Verification items for this drawing (mm, ordinates from the low corner). Coordinates: 2 decimals unless noted, no trailing zeros. Write each loop counter-clockwise with the first axis right and the second up, starting at its lowest first coordinate (ties: lowest second). Pieces come first, ordered by that corner, then holes. Notation, with made-up numbers: (-31.75, 45.5) -> (-10.75, 45.5) arc R18 ccw to (-10.75, 60.5) -> close; hole circle Ø9 at (45, 57). An arc over 180 degrees is marked (long way). Use CSV: the item, a comma, the result in double quotes.
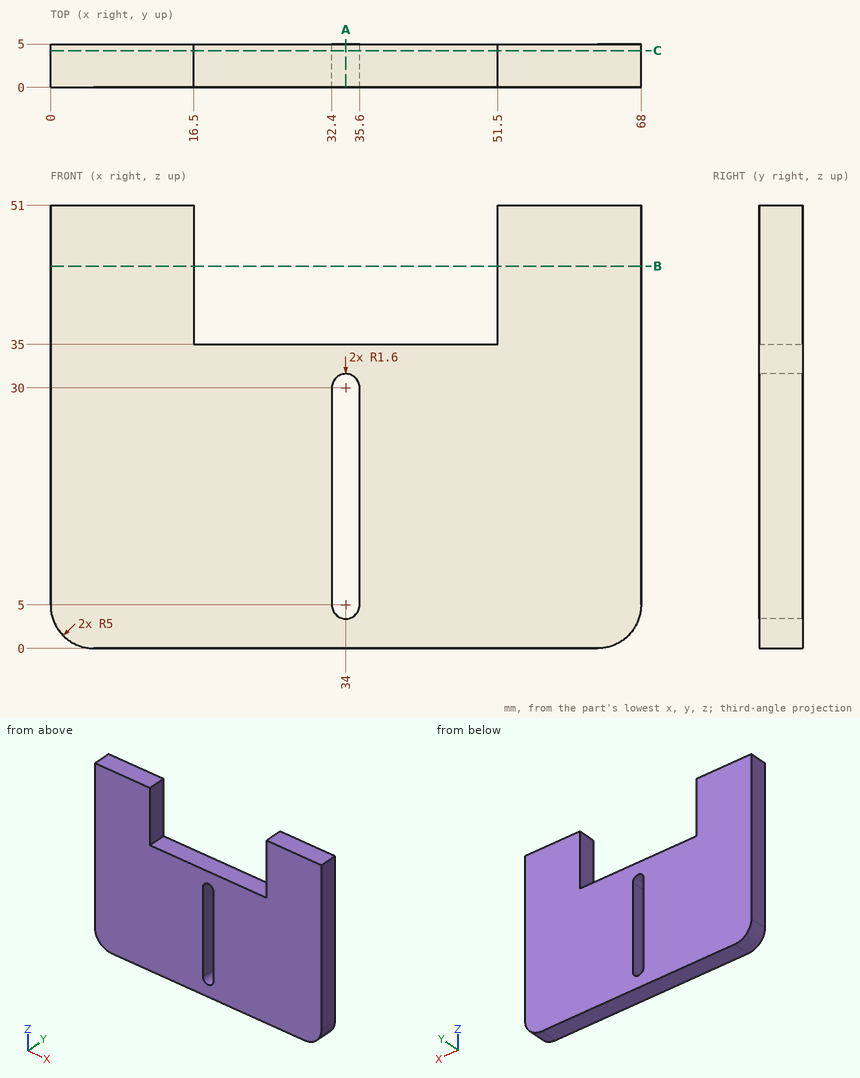
1) Cross-section at B-B (z = 44). Record the boundary of the cut face in (x, y).
Return value:
outline,"(0, 0) -> (16.5, 0) -> (16.5, 5) -> (0, 5) -> close; (51.5, 0) -> (68, 0) -> (68, 5) -> (51.5, 5) -> close"
2) Scan lines: L1, parallel to X at y = 4.05, z = 6.5; L2, parallel to X at y = 3.6, z = 36.5; L3, parallel to Z at x = 17, y = 4.8. Record each from-to range of solid material in increasing order.
Return value:
L1,"0 to 32.4, 35.6 to 68"
L2,"0 to 16.5, 51.5 to 68"
L3,"0 to 35"
3) Cross-section at A-A (x = 34). Record the boundary of the cut face in (y, z).
Return value:
outline,"(0, 0) -> (5, 0) -> (5, 3.4) -> (0, 3.4) -> close; (0, 31.6) -> (5, 31.6) -> (5, 35) -> (0, 35) -> close"
4) Gauge pin test, flat ends, axial feed: pin 1 (6 mm diameter, centred on x = 46, z = 38.5, fed in from +Y); pin 2 (2.5 mm diameter, centred on x = 42, y = 2, fed in from +Z). Record the tip position at first contact, or that the pin passes through.
Return value:
pin 1,"through"
pin 2,"z = 35"
5) Cross-section at C-C (y = 4.25). Record the boundary of the cut face in (x, z).
Return value:
outline,"(0, 5) arc R5 ccw to (5, 0) -> (63, 0) arc R5 ccw to (68, 5) -> (68, 51) -> (51.5, 51) -> (51.5, 35) -> (16.5, 35) -> (16.5, 51) -> (0, 51) -> close; hole (32.4, 5) arc R1.6 ccw to (35.6, 5) -> (35.6, 30) arc R1.6 ccw to (32.4, 30) -> close"
